Verification items for the finished model (mm, model axes). A direction names the side the tool comes from. Round coordinates to 2 decimals unless told otherwise and drop trailing zeros. Write each question's results on one line, items separated by ' | '.
```python
from build123d import *

# Parameters (mm, degrees)
F0_W     = 800.1
F0_H     = 101.6
F1_DEPTH = 101.6
F3_DEPTH = 101.601


with BuildPart() as f1:
    # F0 (on Front) → F1 (new body)
    with BuildSketch(Plane.XZ):
        Rectangle(F0_W, F0_H)
    extrude(amount=F1_DEPTH)

    # F2 (on face) → F3 (cut, through all)
    with BuildSketch(Plane.XZ.offset(101.6)):
        Polygon((12.7, 38.1), (12.7, 63.5), (-12.7, 63.5), (-12.7, 38.1), (0, 38.1), align=None)
    extrude(amount=-F3_DEPTH, mode=Mode.SUBTRACT)


solid = f1.part
```
(1) Go/stop test with flat-tipped pins: pin 1 Ø4 at (x, z) = (-46, -39) entering from +Y; pin 2 Ø20.5 at (x, y) = (2, -61) entering from +Z. Record where each tip stops, or that it passes through.
Answer:
pin 1: y = 0 | pin 2: z = 38.1
(2) Mould release check, pull along X, two halves, no side actions. Record for faces 1 (the flat face through (400.05, -50, -1)), 2 (the flat face through (-6, -101.6, 1)), 3 (the flat face through (-12.7, -52, 45)): released by +X, released by -X, zero draft, split by the parting line, or undercut.
Answer:
face 1: released by +X | face 2: zero draft | face 3: undercut
(3) Thickness scan on L1, parallel to Z at x = -4, y = -49.5. Record the ranges inside material, lowest first.
Answer:
L1: -50.8 to 38.1
(4) Set-up check for faces 4 (the flat face through (-6, 0, 1)), 5 (the flat face through (12.7, -52, 44)): record each of +Z, -Z, +X, -X, +Y, -Y from which the full face is reachable in a straight line by a thin tool's end or side.
Answer:
face 4: +Z, -Z, +X, -X, +Y | face 5: +Z, +Y, -Y
